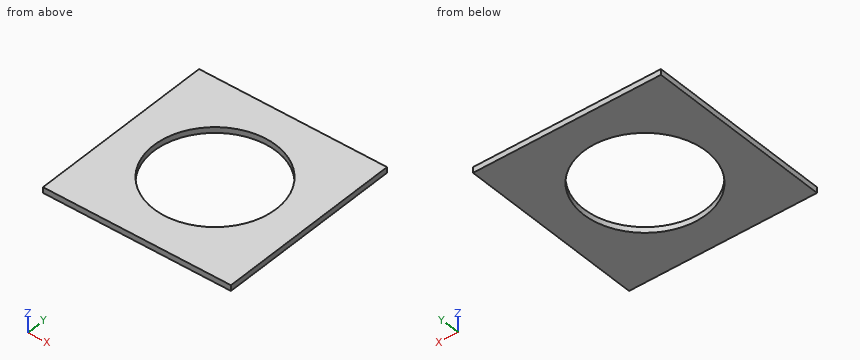
```python
from build123d import *

# Parameters (mm, degrees)
SKETCH1_W           = 330
SKETCH1_H           = 330
BOSS_EXTRUDE1_DEPTH = 10
SKETCH2_R           = 107.5
CUT_EXTRUDE1_DEPTH  = 10


with BuildPart() as part:
    # Sketch1 → Boss-Extrude1 (new body)
    with BuildSketch(Plane.XY):
        Rectangle(SKETCH1_W, SKETCH1_H)
    extrude(amount=-BOSS_EXTRUDE1_DEPTH)

    # Sketch2 → Cut-Extrude1 (cut)
    with BuildSketch(Plane.XY):
        Circle(SKETCH2_R)
    extrude(amount=-CUT_EXTRUDE1_DEPTH, mode=Mode.SUBTRACT)


solid = part.part
```
Could you check a few things on this model? Use its own coordinates, in mm. Coordinates: 2 decimals unless noted, no trailing zeros. Loops run counter-clockwise (first coordinate to the right, second up) from the corner with the lowest first, then second, coordinate; pieces in that order, holes last. Notation, with made-up numbers: M 42.25,-2.75 L 52.25,-2.75 A12 cw 52.25,11.25 Z; hole C 32.25,73 d1. An arc over 180 degrees is marked long. Put each result on its own line as item: value. Start each with the question number.
(1) I need wall thicknesses on line 1 (Y direction, x = 0, z = -4.5); line 2 (Y direction, x = -31.5, z = -6.75); line 3 (X direction, y = -14.5, z = -8.5). Which ranges of each line are inside material? Lowest first, please. Write a range as from..to.
(2) Suppose I cut it at A-A on x = 0. Please give me the cut outline in (y, z), then the cut area to 3 significant figures.
(3) Suppose I cut it at C-C on z = -4.25. Please give me the cut outline in (x, y), then the cut area to 3 significant figures.
Solutions:
1. line 1: y = -165..-107.5, 107.5..165
1. line 2: y = -165..-102.78, 102.78..165
1. line 3: x = -165..-106.52, 106.52..165
2. outline: M -165,-10 L -107.5,-10 L -107.5,0 L -165,0 Z; M 107.5,-10 L 165,-10 L 165,0 L 107.5,0 Z
2. area: 1,150 mm2
3. outline: M -165,-165 L 165,-165 L 165,165 L -165,165 Z; hole C 0,0 d215
3. area: 72,600 mm2
